Design review of the part built by this model. Coordinates are the model's own, in mm. Face numbers are marked on the shaded views. Give positions to 0.01 mm unless a question says otherwise; leave off trailing zeros. Write each loop counter-clockwise with the first axis right and the second up, starting at its lowest first coordinate (ties: lowest second). Pieces come first, ordered by that corner, then holes.
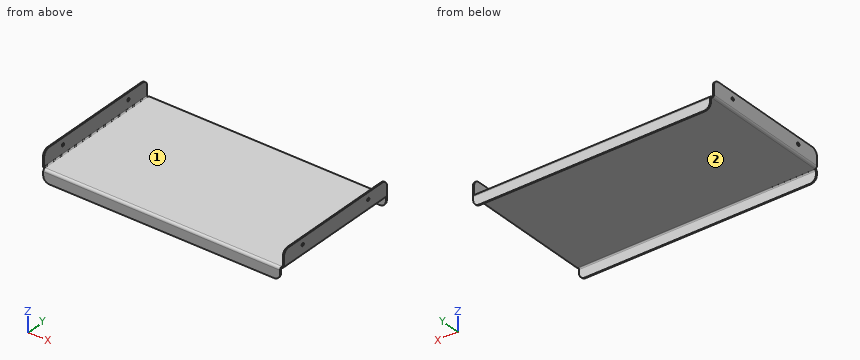
```python
from build123d import *

# Parameters (mm, degrees)
SKETCH1_W                    = 200
SKETCH1_H                    = 110
BASE_FLANGE1_DEPTH           = 1
EDGE_FLANGE1_STRIP_W         = 5.4732
EDGE_FLANGE1_STRIP_H         = 1
EDGE_FLANGE1_STRIP_CUT_DEPTH = 110
EDGE_FLANGE1_DEPTH           = 110
EDGE_FLANGE2_STRIP_W         = 5.4732
EDGE_FLANGE2_STRIP_H         = 1
EDGE_FLANGE2_STRIP_CUT_DEPTH = 110
EDGE_FLANGE2_DEPTH           = 110
CUT_EXTRUDE1_DEPTH           = 207.869524097
CUT_EXTRUDE1_DEPTH_BACK      = 10
SKETCH14_R                   = 1.25
EDGE_FLANGE3_DEPTH           = 196.5268
EDGE_FLANGE3_BEND_DEPTH      = 196.5268
FILLET1_R                    = 5


# Sheet-metal steps are written as plain solids
with BuildPart() as part:
    # Sketch1 → Base-Flange1 (new body)
    with BuildSketch(Plane.XY):
        Rectangle(SKETCH1_W, SKETCH1_H)
    extrude(amount=-BASE_FLANGE1_DEPTH)

    # Edge-Flange1 strip (across the edge) → Edge-Flange1 strip cut (cut)
    with BuildSketch(Plane(origin=(-100, 55, 0), x_dir=(1, 0, 0), z_dir=(0, -1, 0))):
        with Locations((-1, -0.5)):
            Rectangle(EDGE_FLANGE1_STRIP_W, EDGE_FLANGE1_STRIP_H)
    extrude(amount=EDGE_FLANGE1_STRIP_CUT_DEPTH, mode=Mode.SUBTRACT)

    # Edge-Flange1 section (across the edge) → Edge-Flange1 (add)
    with BuildSketch(Plane(origin=(-100, 55, 0), x_dir=(1, 0, 0), z_dir=(0, -1, 0))):
        with BuildLine():
            Line((0, 0.7366), (0, 13))
            Line((0, 13), (1, 13))
            Line((1, 13), (1, 0.7366))
            ThreePointArc((1, 0.7366), (1.215745145, 0.215745145), (1.7366, 0))
            Line((1.7366, 0), (1.7366, -1))
            ThreePointArc((1.7366, -1), (0.508638364, -0.491361636), (0, 0.7366))
        make_face()
    extrude(amount=EDGE_FLANGE1_DEPTH)

    # Edge-Flange2 strip (across the edge) → Edge-Flange2 strip cut (cut)
    with BuildSketch(Plane(origin=(100, -55, 0), x_dir=(-1, 0, 0), z_dir=(0, 1, 0))):
        with Locations((-1, -0.5)):
            Rectangle(EDGE_FLANGE2_STRIP_W, EDGE_FLANGE2_STRIP_H)
    extrude(amount=EDGE_FLANGE2_STRIP_CUT_DEPTH, mode=Mode.SUBTRACT)

    # Edge-Flange2 section (across the edge) → Edge-Flange2 (add)
    with BuildSketch(Plane(origin=(100, -55, 0), x_dir=(-1, 0, 0), z_dir=(0, 1, 0))):
        with BuildLine():
            Line((0, 0.7366), (0, 13))
            Line((0, 13), (1, 13))
            Line((1, 13), (1, 0.7366))
            ThreePointArc((1, 0.7366), (1.215745145, 0.215745145), (1.7366, 0))
            Line((1.7366, 0), (1.7366, -1))
            ThreePointArc((1.7366, -1), (0.508638364, -0.491361636), (0, 0.7366))
        make_face()
    extrude(amount=EDGE_FLANGE2_DEPTH)

    # Sketch14 → Cut-Extrude1 (cut, two sides: drawn at the far end of the back side and taken through both)
    with BuildSketch(Plane(origin=(-99, 0, 0), x_dir=(0, 0, -1), z_dir=(1, 0, 0)).offset(-CUT_EXTRUDE1_DEPTH_BACK)):
        with Locations(Location((-7.5, -35, 0), (0, 0, 180))):
            Circle(SKETCH14_R)
        with Locations(Location((-7.5, 35, 0), (0, 0, 180))):
            Circle(SKETCH14_R)
    extrude(amount=CUT_EXTRUDE1_DEPTH + CUT_EXTRUDE1_DEPTH_BACK, mode=Mode.SUBTRACT)

    # Edge-Flange3 section (across the edge) → Edge-Flange3 (add)
    with BuildSketch(Plane(origin=(98.2634, -56, -1), x_dir=(0, 1, 0), z_dir=(-1, 0, 0))):
        with BuildLine():
            Line((-1, 1), (-1, 9))
            Line((-1, 9), (0, 9))
            Line((0, 9), (0, 1))
            ThreePointArc((0, 1), (0.292893219, 0.292893219), (1, 0))
            Line((1, 0), (1, -1))
            ThreePointArc((1, -1), (-0.414213562, -0.414213562), (-1, 1))
        make_face()
    extrude(amount=EDGE_FLANGE3_DEPTH)

    # Edge-Flange3 section 2 (across the edge) → Edge-Flange3 bend (add)
    with BuildSketch(Plane(origin=(-98.2634, 56, -1), x_dir=(0, -1, 0), z_dir=(1, 0, 0))):
        with BuildLine():
            Line((-1, 1), (-1, 9))
            Line((-1, 9), (0, 9))
            Line((0, 9), (0, 1))
            ThreePointArc((0, 1), (0.292893219, 0.292893219), (1, 0))
            Line((1, 0), (1, -1))
            ThreePointArc((1, -1), (-0.414213562, -0.414213562), (-1, 1))
        make_face()
    extrude(amount=EDGE_FLANGE3_BEND_DEPTH)

    # Fillet1
    fillet1_edges = [part.edges().sort_by_distance(p)[0] for p in [
        (98.2634, -56.5, -10),
        (-98.2634, -56.5, -10),
        (-98.2634, 56.5, -10),
        (98.2634, 56.5, -10),
        (-99.5, 55, 13),
        (-99.5, -55, 13),
        (99.5, -55, 13),
        (99.5, 55, 13),
    ]]
    fillet(fillet1_edges, radius=FILLET1_R)


solid = part.part
```
(1) Mouldability with a two-part tool opening along X and no side actions: class the marked faces 1 and 2 as pulls with the +X half, pulls with the -X half, needs draft (parallel to the pull), parting line crosses it, or undercut.
Resolved:
face 1: undercut
face 2: needs draft
(2) Consider section B-B, the plane y = 5.5. Give the boundary of the cut face in (x, z), then the cut area to 3 significant figures.
Resolved:
outline: (-100, 0.74) arc R1.74 ccw to (-98.26, -1) - (98.26, -1) arc R1.74 ccw to (100, 0.74) - (100, 13) - (99, 13) - (99, 0.74) arc R0.74 cw to (98.26, 0) - (-98.26, 0) arc R0.74 cw to (-99, 0.74) - (-99, 13) - (-100, 13) - close
area: 225 mm2
(3) Clearance check with flat-ended pins moving along their axes: P1, Ø1.6, axis at y = -56, z = -2, coming from the +X side; P2, Ø0.9, axis at x = 99.5, z = 2, coming from the +Y side; P3, Ø5, axis at x = 27, y = -20.5, coming from the +Z side. State where each tip first meets the part, or that it passes through.
Resolved:
P1: stops at x = 98.26
P2: stops at y = 55
P3: stops at z = 0
(4) To check wall thickness, follow L1, parallel to Y at x = -99.5, z = 7.5; L2, parallel to X at y = -9, z = 7.5; L3, parallel to Z at x = 33.5, y = -40. State the ranges of each line that lie inside material, in increasing order.
Resolved:
L1: y = -55 to -36.25, -33.75 to 33.75, 36.25 to 55
L2: x = -100 to -99, 99 to 100
L3: z = -1 to 0
(5) Consider section A-A, the plane x = 77. Give the boundary of the cut face in (y, z), then the cut area to 3 significant figures.
Resolved:
outline: (-57, -10) - (-56, -10) - (-56, -2) arc R1 cw to (-55, -1) - (55, -1) arc R1 cw to (56, -2) - (56, -10) - (57, -10) - (57, -2) arc R2 ccw to (55, 0) - (-55, 0) arc R2 ccw to (-57, -2) - close
area: 131 mm2
